Verification items for the finished model (mm, model axes). A direction names the side the tool comes from. Round coordinates to 2 decimals unless told otherwise and drop trailing zeros. Loops run counter-clockwise (first coordinate to the right, second up) from the corner with the lowest first, then second, coordinate; pieces in that order, holes last. Notation, with made-up numbers: (-3.5, -25.5) -> (25.5, -25.5) arc R17 cw to (25.5, 6.5) -> close; hole circle Ø11 at (-35, 58.5). An arc over 180 degrees is marked (long way). Use a Markdown table: item, result. Add a question column.
```python
from build123d import *

# Parameters (mm, degrees)
SKETCH1_R           = 2.5
BOSS_EXTRUDE1_DEPTH = 250
FILLET1_R           = 1
FILLET2_R           = 0.5
FILLET3_R           = 0.5
FILLET4_R           = 0.5
FILLET5_R           = 0.5
CUT_EXTRUDE3_DEPTH  = 252.594912508
CUT_EXTRUDE5_DEPTH  = 252.594912508


with BuildPart() as part:
    # Sketch1 → Boss-Extrude1 (new body)
    with BuildSketch(Plane.XY):
        Polygon((13.2, 0), (13.2, 1.8), (15.45, 1.8), (15.45, 3.6), (12.95, 6.1), (7.05, 6.1), (4.55, 3.6), (4.55, 1.8), (6.8, 1.8), (6.8, 0), (0, 0), (0, 6.8), (1.8, 6.8), (1.8, 4.55), (3.6, 4.55), (6.1, 7.05), (6.1, 12.95), (3.6, 15.45), (1.8, 15.45), (1.8, 13.2), (0, 13.2), (0, 20), (6.8, 20), (6.8, 18.2), (4.55, 18.2), (4.55, 16.4), (7.05, 13.9), (12.95, 13.9), (15.45, 16.4), (15.45, 18.2), (13.2, 18.2), (13.2, 20), (20, 20), (20, 13.2), (18.2, 13.2), (18.2, 15.45), (16.4, 15.45), (13.9, 12.95), (13.9, 7.05), (16.4, 4.55), (18.2, 4.55), (18.2, 6.8), (20, 6.8), (20, 0), align=None)
        with Locations((10, 10)):
            Circle(SKETCH1_R, mode=Mode.SUBTRACT)
    extrude(amount=BOSS_EXTRUDE1_DEPTH)

    # Fillet1
    fillet1_edges = [part.edges().sort_by_distance(p)[0] for p in [
        (0, 0, 125),
        (0, 20, 125),
        (20, 20, 125),
        (20, 0, 125),
    ]]
    fillet(fillet1_edges, radius=FILLET1_R)

    # Fillet2
    fillet2_edges = [part.edges().sort_by_distance(p)[0] for p in [
        (4.55, 18.2, 125),
        (4.55, 16.4, 125),
        (7.05, 13.9, 125),
        (12.95, 13.9, 125),
        (15.45, 16.4, 125),
        (15.45, 18.2, 125),
    ]]
    fillet(fillet2_edges, radius=FILLET2_R)

    # Fillet3
    fillet3_edges = [part.edges().sort_by_distance(p)[0] for p in [
        (18.2, 15.45, 125),
        (16.4, 15.45, 125),
        (13.9, 12.95, 125),
        (13.9, 7.05, 125),
        (16.4, 4.55, 125),
        (18.2, 4.55, 125),
    ]]
    fillet(fillet3_edges, radius=FILLET3_R)

    # Fillet4
    fillet4_edges = [part.edges().sort_by_distance(p)[0] for p in [
        (1.8, 4.55, 125),
        (3.6, 4.55, 125),
        (6.1, 7.05, 125),
        (6.1, 12.95, 125),
        (3.6, 15.45, 125),
        (1.8, 15.45, 125),
    ]]
    fillet(fillet4_edges, radius=FILLET4_R)

    # Fillet5
    fillet5_edges = [part.edges().sort_by_distance(p)[0] for p in [
        (15.45, 1.8, 125),
        (15.45, 3.6, 125),
        (12.95, 6.1, 125),
        (7.05, 6.1, 125),
        (4.55, 3.6, 125),
        (4.55, 1.8, 125),
    ]]
    fillet(fillet5_edges, radius=FILLET5_R)

    # Sketch4 → Cut-Extrude3 (cut, through all)
    with BuildSketch(Plane.XZ):
        Polygon((20, 250), (20, 215.358983849), (0, 250), align=None)
    extrude(amount=-CUT_EXTRUDE3_DEPTH, mode=Mode.SUBTRACT)

    # Sketch6 → Cut-Extrude5 (cut, through all)
    with BuildSketch(Plane.XZ):
        Polygon((20, 0), (0, 0), (20, 34.641016151), align=None)
    extrude(amount=-CUT_EXTRUDE5_DEPTH, mode=Mode.SUBTRACT)


solid = part.part
```
1) Sectioned sample at B-B on x = 10. Enter the section's corners in (y, z), then the cut area to 3 significant figures.
2) Sectioned sample at A-A on y = 10. Enter the section's corners in (x, z), then the cut area to 3 significant figures.
3) Access from +Z, -Z, +X, -X, +Y, -Y to the whole of each face (thin tool, end or side, straight path). Record for faces 5 (the face through (10, 13.9, 123)), 6 (the face through (13.9, 10, 124)), 7 (the face through (16, 0, 124)).
4) Release check for a two-part mould opening along X. For faces 1 (the face through (20, 16, 124)), 2 (the face through (10, 6.1, 123)), 3 (the face through (6.1, 10, 123)), 4 (the face through (16, 20, 124)) record: released by +X, released by -X, zero draft, split by the parting line, or undercut.
5) Go/stop test with flat-tipped pins: pin 1 (4.5 mm diameter, centred on y = 9.5, z = 75.5, fed in from -X); pin 2 (3 mm diameter, centred on x = 5, y = 16, fed in from -Z); pin 3 (1.5 mm diameter, centred on x = 7.5, y = 9.5, fed in from -Z). Record where each tip stops, or that it passes through.
6) Thickness scan on line 1 (X direction, y = 10, z = 163); line 2 (X direction, y = 17.5, z = 154). Record the ranges inside material, lowest first.
Geometry results:
| question | item | result |
|---|---|---|
| 1 | outline | (6.1, 17.32) -> (7.5, 17.32) -> (7.5, 232.68) -> (6.1, 232.68) -> close; (12.5, 17.32) -> (13.9, 17.32) -> (13.9, 232.68) -> (12.5, 232.68) -> close |
| 1 | area | 603 mm^2 |
| 2 | outline | (6.1, 10.57) -> (7.5, 12.99) -> (7.5, 237.01) -> (6.1, 239.43) -> close; (12.5, 21.65) -> (13.9, 24.08) -> (13.9, 225.92) -> (12.5, 228.35) -> close |
| 2 | area | 603 mm^2 |
| 3 | face 5 | +Z, -Z, +Y |
| 3 | face 6 | +Z, -Z, +X |
| 3 | face 7 | +Z, -Z, +X, -X, -Y |
| 4 | face 1 | released by +X |
| 4 | face 2 | undercut |
| 4 | face 3 | released by -X |
| 4 | face 4 | zero draft |
| 5 | pin 1 | x = 6.1 |
| 5 | pin 2 | z = 6.06 |
| 5 | pin 3 | z = 11.69 |
| 6 | line 1 | 6.1 to 7.5, 12.5 to 13.9 |
| 6 | line 2 | 0 to 4.55, 15.45 to 20 |
